```python
from build123d import *

# Parameters (mm, degrees)
F1_DEPTH = 50.8
F3_DEPTH = 50.8


with BuildPart() as f1:
    # F0 (on Front) → F1 (new body)
    with BuildSketch(Plane.XZ):
        Polygon((-50.8, 0), (0, 0), (0, 38.1), (-25.4, 38.1), (-25.4, 63.5), (-50.8, 63.5), align=None)
    extrude(amount=F1_DEPTH)

    # F2 (on face) → F3 (cut)
    with BuildSketch(Plane.XZ.offset(50.8)):
        with BuildLine():
            Line((-25.4, 38.1), (-25.4, 63.5))
            ThreePointArc((-25.4, 63.5), (-24.36322, 33.245019), (0, 15.276372))
            Line((0, 15.276372), (0, 38.1))
            Line((0, 38.1), (-25.4, 38.1))
        make_face()
    extrude(amount=-F3_DEPTH, mode=Mode.SUBTRACT)


solid = f1.part
```
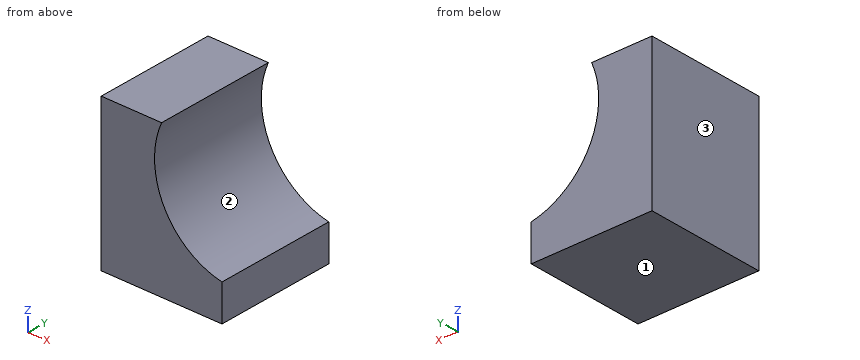
Geometry check sheet. Reference: the model listing, model coordinates, mm. Face numbers are marked on the shaded views. Coordinates: 2 decimals unless noted, no trailing zeros. Loops run counter-clockwise (first coordinate to the right, second up) from the corner with the lowest first, then second, coordinate; pieces in that order, holes last. Notation, with made-up numbers: (28, -10.75) - (38, -10.75) arc R20 cw to (38, 14.25) - close; hole circle Ø1 at (-33, -15). An arc over 180 degrees is marked (long way). One line per item, written item: value. Start each with the question number.
(1) Cross-section at A-A on y = -15.5. Enter the section's corners in (x, z).
(2) Cross-section at C-C on x = -15. Enter the section's corners in (y, z), plus the area to 3 significant figures.
(3) Material ranges on line 1 (X direction, y = -25, z = 50); line 2 (Z direction, x = -13, y = -40); line 3 (Z direction, x = -5.5, y = -28.5), recorded low to high. Write a range as [from, to].
(4) Cross-section at B-B on z = 26. Enter the section's corners in (x, y).
(5) Mould release check, pull along Z, two halves, no side actions. Record for the marked faces 1, 2 and 3: released by +Z, released by -Z, zero draft, split by the parting line, or undercut.
(6) Depth check by flat-ended pin: P1, Ø5, axis at x = -33, y = -45, coming from the -Z side; P2, Ø12, axis at x = -16.5, y = -8, coming from the +Z side; P3, Ø1, axis at x = -18.5, y = -20.5, coming from the +Z side; P4, Ø1, axis at x = -19, y = -18, coming from the +Z side. Enter the tip coordinate at first touch or a pass-through.
Results below:
1. outline: (-50.8, 0) - (0, 0) - (0, 15.28) arc R34.76 cw to (-25.4, 63.5) - (-50.8, 63.5) - close
2. outline: (-50.8, 0) - (0, 0) - (0, 22.05) - (-50.8, 22.05) - close
2. area: 1,120 mm2
3. line 1: x = [-50.8, -28.36]
3. line 2: z = [0, 20.6]
3. line 3: z = [0, 16.78]
4. outline: (-50.8, -50.8) - (-19.27, -50.8) - (-19.27, 0) - (-50.8, 0) - close
5. face 1: released by -Z
5. face 2: undercut
5. face 3: zero draft
6. P1: stops at z = 0
6. P2: stops at z = 30.12
6. P3: stops at z = 25.71
6. P4: stops at z = 26.25
